Check sheet for the modelled part. Datum: model origin and axes. Units: mm. A direction names the side the tool comes from. Round coordinates to 2 decimals unless told otherwise and drop trailing zeros. Order: outer loops, then holes, each group sorted by start corner. A loop starts at its lowest first (then second) coordinate and runs counter-clockwise, first axis right, second up. Notation, with made-up numbers: (63.5, -34) -> (71.5, -34) arc R19 cw to (71.5, -30) -> close; hole circle Ø6 at (38, 30). An arc over 180 degrees is marked (long way). Use CSV: the item, a comma, the result in double quotes.
```python
from build123d import *

# Parameters (mm, degrees)
F0_W     = 2032
F0_H     = 1016
F1_DEPTH = 635
F2_W     = 1016
F2_H     = 711.2
F3_DEPTH = 381
F4_W     = 508
F4_H     = 508
F5_DEPTH = 381


with BuildPart() as f1:
    # F0 (on Top) → F1 (new body)
    with BuildSketch(Plane.XY):
        with Locations((-18.151204, -1410.432026)):
            Rectangle(F0_W, F0_H)
    extrude(amount=F1_DEPTH)

    # F2 (on face) → F3 (join)
    with BuildSketch(Plane(origin=(0, 0, 0), x_dir=(1, 0, 0), z_dir=(0, 0, -1))):
        with Locations((489.848796, 1562.832026)):
            Rectangle(F2_W, F2_H)
    extrude(amount=F3_DEPTH)

    # F4 (on face) → F5 (cut)
    with BuildSketch(Plane(origin=(0, 0, 0), x_dir=(1, 0, 0), z_dir=(0, 0, -1))):
        with Locations((-780.151204, 1156.432026)):
            Rectangle(F4_W, F4_H)
    extrude(amount=-F5_DEPTH, mode=Mode.SUBTRACT)


solid = f1.part
```
Q1. Sectioned sample at A-A, the plane z = 305.5. Enter the section's corners in (x, y).
Result sheet:
outline,"(-1034.15, -1918.43) -> (997.85, -1918.43) -> (997.85, -902.43) -> (-526.15, -902.43) -> (-526.15, -1410.43) -> (-1034.15, -1410.43) -> close"
Q2. Access from +Z, -Z, +X, -X, +Y, -Y to the whole of each face (thin tool, end or side, straight path). Record for faces 1 (the face through (-18.151, -1558, -188)), 2 (the face through (483, -1207.232, -188)), 3 (the face through (483, -1568, -381)), 4 (the face through (-1034.151, -1530, 384)), 5 (the face through (-526.151, -1153, 188)).
Result sheet:
face 1,"-Z, -X, +Y, -Y"
face 2,"-Z, +X, -X, +Y"
face 3,"-Z, +X, -X, +Y, -Y"
face 4,"+Z, -Z, -X, +Y, -Y"
face 5,"-Z, -X, +Y"
Q3. Sectioned sample at C-C, the plane x = -136. Enter the section's corners in (y, z), then the cut area to 3 significant figures.
Result sheet:
outline,"(-1918.43, 0) -> (-902.43, 0) -> (-902.43, 635) -> (-1918.43, 635) -> close"
area,"645,000 mm^2"
Q4. Go/stop test with flat-tipped pins: pin 1 (3 mm diameter, centred on x = -369, y = -1236.5, fed in from -Z); pin 2 (1.5 mm diameter, centred on y = -1465.5, z = -104.5, fed in from -X). Record where each tip stops, or that it passes through.
Result sheet:
pin 1,"stops at z = 0"
pin 2,"stops at x = -18.15"
Q5. Sectioned sample at B-B, the plane y = -1112. Enter the section's corners in (x, z), then the cut area to 3 significant figures.
Result sheet:
outline,"(-1034.15, 381) -> (-526.15, 381) -> (-526.15, 0) -> (997.85, 0) -> (997.85, 635) -> (-1034.15, 635) -> close"
area,"1,100,000 mm^2"
Q6. Scan lines: L1, parallel to Z at x = -681.5, y = -1009.5; L2, parallel to X at y = -1791.5, z = -250; L3, parallel to X at y = -1230.5, z = 31. Record each from-to range of solid material in increasing order.
Result sheet:
L1,"z = 381 to 635"
L2,"x = -18.15 to 997.85"
L3,"x = -526.15 to 997.85"
Q7. Sectioned sample at D-D, the plane z = -42. Enter the section's corners in (x, y).
Result sheet:
outline,"(-18.15, -1918.43) -> (997.85, -1918.43) -> (997.85, -1207.23) -> (-18.15, -1207.23) -> close"
